Design review of the part built by this model. Coordinates are the model's own, in mm. A direction names the side the tool comes from. Coordinates: 2 decimals unless noted, no trailing zeros. Loops run counter-clockwise (first coordinate to the right, second up) from the corner with the lowest first, then second, coordinate; pieces in that order, holes last. Notation, with made-up numbers: M 23,-17.5 L 56,-17.5 A36 cw 56,19.5 Z; hole C 83,22 d8. An arc over 180 degrees is marked long. Put each result on its own line as item: value. Start each with the question number.
(1) For faces 1 (the cylindrical face through (1.288, -25.953, 80.058)), 2 (the flat face through (22.86, -36, 63)), list the 3-axis set-ups (+Z, -Z, +X, -X, +Y, -Y) from which the entire face can be reached by the end or side of a thin tool; tool diameter is ignored.
(2) Take a section at C-C, the plane z = 26.5. Give the boundary of the cut face in (x, y), then the cut area to 3 significant figures.
(3) Take a section at D-D, the plane y = -25.4. Count the separate pieces of the cut face and the enclosed holes in it, then the cut area to 3 significant figures.
(4) Take a section at A-A, the plane x = 6.75. Give the boundary of the cut face in (y, z).
(5) For probe 1 along Z at (x, y) = (1.45, -25.4); probe 2 along X at (y, z) = (-27, 117); probe 3 along Y at (x, z) = (10, 71.5), list the stretches that pass through material, from the lowest coordinate up. Write a range as [from, to].
(6) The part is to be moulded in two halves that separate along X. For faces 3 (the flat face through (0, -37, 63)), 4 (the flat face through (13, 0, 63)), 5 (the flat face through (13, -48.26, 63)), say which applies: +X half, -X half, draft (parallel to the pull), parting line (faces both ways), or undercut.
(7) Take a section at B-B, the plane z = 82.55. Give the boundary of the cut face in (x, y).
```python
from build123d import *

# Parameters (mm, degrees)
F0_W     = 25.4
F0_H     = 50.8
F0_W_2   = 20.32
F0_H_2   = 45.72
F1_DEPTH = 127
F2_R     = 2.5527
F2_R_2   = 14.2875
F3_DEPTH = 50.8


# Not quite as in the source:
# - a feature names something its author has since deleted; it is built from what else it names


with BuildPart() as f1:
    # F0 (on Top) → F1 (new body)
    with BuildSketch(Plane.XY):
        with Locations((12.7, -25.4)):
            Rectangle(F0_W, F0_H)
        with Locations((12.7, -25.4)):
            Rectangle(F0_W_2, F0_H_2, mode=Mode.SUBTRACT)
    extrude(amount=F1_DEPTH)

    # F2 (on face) → F3 (cut)
    with BuildSketch(Plane.YZ.offset(25.4)):
        with BuildLine():
            ThreePointArc((-43.3605122421, 68.7605122421), (-42.4353064615, 69.6403379418), (-41.467058279, 70.4725605415))
            ThreePointArc((-41.467058279, 70.4725605415), (-45.1655437225, 70.5655437225), (-45.0725605415, 66.867058279))
            ThreePointArc((-45.0725605415, 66.867058279), (-44.2403379418, 67.8353064615), (-43.3605122421, 68.7605122421))
        make_face()
        with Locations((-25.4, 82.55)):
            Circle(F2_R)
        with Locations((-25.4, 12.7)):
            Circle(F2_R)
        with BuildLine():
            Line((-25.4, 50.8), (-15.2972118638, 40.6972118638))
            ThreePointArc((-15.2972118638, 40.6972118638), (-12.2000711792, 45.3324104601), (-11.1125, 50.8))
            ThreePointArc((-11.1125, 50.8), (-19.9324104601, 63.9999288208), (-35.5027881362, 60.9027881362))
            Line((-35.5027881362, 60.9027881362), (-25.4, 50.8))
        make_face()
        with BuildLine():
            Line((-25.4, 50.8), (-35.5027881362, 60.9027881362))
            ThreePointArc((-35.5027881362, 60.9027881362), (-38.5999288208, 56.2675895399), (-39.6875, 50.8))
            Line((-39.6875, 50.8), (-25.4, 50.8))
        make_face()
        with BuildLine():
            Line((-41.5554807618, 66.9554807618), (-43.3605122421, 68.7605122421))
            ThreePointArc((-43.3605122421, 68.7605122421), (-44.2403379418, 67.8353064615), (-45.0725605415, 66.867058279))
            ThreePointArc((-45.0725605415, 66.867058279), (-43.2963553886, 66.2086185946), (-41.5554807618, 66.9554807618))
        make_face()
        with BuildLine():
            ThreePointArc((-40.8078122421, 68.7605122421), (-40.9783181672, 69.6778064584), (-41.467058279, 70.4725605415))
            ThreePointArc((-41.467058279, 70.4725605415), (-42.4353064615, 69.6403379418), (-43.3605122421, 68.7605122421))
            Line((-43.3605122421, 68.7605122421), (-41.5554807618, 66.9554807618))
            ThreePointArc((-41.5554807618, 66.9554807618), (-41.0021249595, 67.7836362443), (-40.8078122421, 68.7605122421))
        make_face()
        with BuildLine():
            ThreePointArc((-39.6875, 50.8), (-30.8675895399, 37.6000711792), (-15.2972118638, 40.6972118638))
            Line((-15.2972118638, 40.6972118638), (-25.4, 50.8))
            Line((-25.4, 50.8), (-39.6875, 50.8))
        make_face()
        with BuildLine():
            ThreePointArc((-4.8867877579, 32.8394877579), (-5.1063972127, 33.8753283817), (-5.7274394585, 34.732941721))
            ThreePointArc((-5.7274394585, 34.732941721), (-6.5596620582, 33.7646935385), (-7.4394877579, 32.8394877579))
            ThreePointArc((-7.4394877579, 32.8394877579), (-8.3646935385, 31.9596620582), (-9.332941721, 31.1274394585))
            ThreePointArc((-9.332941721, 31.1274394585), (-6.5221935416, 30.4572936829), (-4.8867877579, 32.8394877579))
        make_face()
        with BuildLine():
            ThreePointArc((-7.4394877579, 32.8394877579), (-6.5596620582, 33.7646935385), (-5.7274394585, 34.732941721))
            ThreePointArc((-5.7274394585, 34.732941721), (-7.5036446114, 35.3913814054), (-9.2445192382, 34.6445192382))
            Line((-9.2445192382, 34.6445192382), (-7.4394877579, 32.8394877579))
        make_face()
        with BuildLine():
            ThreePointArc((-9.332941721, 31.1274394585), (-8.3646935385, 31.9596620582), (-7.4394877579, 32.8394877579))
            Line((-7.4394877579, 32.8394877579), (-9.2445192382, 34.6445192382))
            ThreePointArc((-9.2445192382, 34.6445192382), (-9.9913814054, 32.9036446114), (-9.332941721, 31.1274394585))
        make_face()
        with Locations((-25.4, 120.65)):
            Circle(F2_R)
        with Locations((-25.4, 101.6)):
            Circle(F2_R_2)
    extrude(amount=-F3_DEPTH, mode=Mode.SUBTRACT)


solid = f1.part
```
Computed values:
1. face 1: +X, -X
1. face 2: +Z, -Z
2. outline: M 0,-50.8 L 25.4,-50.8 L 25.4,0 L 0,0 Z; hole M 2.54,-48.26 L 22.86,-48.26 L 22.86,-2.54 L 2.54,-2.54 Z
2. area: 361 mm^2
3. separate pieces: 12
3. enclosed holes: 0
3. area: 277 mm^2
4. outline: M -50.8,0 L -48.26,0 L -48.26,127 L -50.8,127 Z; M -2.54,0 L 0,0 L 0,127 L -2.54,127 Z
5. probe 1: z = [0, 10.15], [15.25, 36.51], [65.09, 80], [85.1, 87.31], [115.89, 118.1], [123.2, 127]
5. probe 2: x = [0, 2.54], [22.86, 25.4]
5. probe 3: y = [-50.8, -48.26], [-2.54, 0]
6. face 3: -X half
6. face 4: draft
6. face 5: undercut
7. outline: M 0,-50.8 L 25.4,-50.8 L 25.4,-27.95 L 22.86,-27.95 L 22.86,-48.26 L 2.54,-48.26 L 2.54,-27.95 L 0,-27.95 Z; M 0,-22.85 L 2.54,-22.85 L 2.54,-2.54 L 22.86,-2.54 L 22.86,-22.85 L 25.4,-22.85 L 25.4,0 L 0,0 Z
